Geometry: final body of the model. Coordinates: model frame, mm. Face numbers are marked on the shaded views. A direction names the side the tool comes from. Coordinates: 2 decimals unless noted, no trailing zeros. Loops run counter-clockwise (first coordinate to the right, second up) from the corner with the lowest first, then second, coordinate; pieces in that order, holes last. Notation, with made-up numbers: (74.5, 46) -> (111.5, 46) arc R21 cw to (111.5, 51) -> close; hole circle Ø9 at (28, -8). An arc over 180 degrees is marked (long way). One line per item, written item: value. Start each with the question number.
Item 1: Section query A-A on y = -14. Return loops of the section in (x, z), then the cut area to 3 significant figures.
Item 2: Section query C-C on z = 11.5. Return loops of the section in (x, y).
Item 3: Ray query, probe 1 along Y at (x, z) = (0, 1); probe 2 along Z at (x, y) = (-55.5, -6.5); probe 3 along Y at (x, z) = (0, 27). Return the intervals inside material, ascending. Write a range as from..to.
Item 4: Section query D-D on z = 34.5. Return loops of the section in (x, y), then the cut area to 3 significant figures.
Item 5: Mould query, pull axis Y, two halves, no side actions, for the marked faces 1, 2, 3 and 4. Classes: +Y half, -Y half, draft (parallel to the pull), parting line (faces both ways), or undercut.
Item 6: Set-up query: the marked faces 5, 6 and 7. Return all of +Z, -Z, +X, -X, +Y, -Y with unobstructed straight access to the full face (end or side cutting, diameter ignored); none if empty.
Item 7: Section query B-B on x = -10.5. Return loops of the section in (y, z).
Item 8: Contact query for flat-ended pins moving along their axis: pin 1 Ø12 at (y, z) = (-17, 18.5) entering from +X; pin 2 Ø19.5 at (x, z) = (-60, 18) entering from -Y; pin 3 Ø12 at (x, y) = (50, -44.5) entering from +Z; pin 4 Ø7.5 at (x, z) = (59, 16) entering from -Y. Output: stop coordinate, or through.
from build123d import *

# Parameters (mm, degrees)
F0_R      = 67.5
F1_DEPTH  = 3
F2_R      = 43
F2_R_2    = 41
F3_DEPTH  = 35
F4_R      = 27.5
F5_DEPTH  = 3
F7_DEPTH  = 25
F12_DEPTH = 25
F13_DEPTH = 25
F14_DEPTH = 25
F15_DEPTH = 25
F16_DEPTH = 25


with BuildPart() as f1:
    # F0 (on Top) → F1 (new body)
    with BuildSketch(Plane.XY):
        Circle(F0_R)
    extrude(amount=F1_DEPTH)

    # F2 (on face) → F3 (join)
    with BuildSketch(Plane.XY.offset(3)):
        Circle(F2_R)
        Circle(F2_R_2, mode=Mode.SUBTRACT)
    extrude(amount=F3_DEPTH)

    # F4 (on face) → F5 (cut)
    with BuildSketch(Plane.XY.offset(3)):
        Circle(F4_R)
    extrude(amount=-F5_DEPTH, mode=Mode.SUBTRACT)

    # F6 (on face) → F7 (join)
    with BuildSketch(Plane.XY.offset(3)):
        with BuildLine():
            ThreePointArc((-1.4872706737, -67.4836130179), (0.0127324705, -67.4999987991), (1.5127293263, -67.4830471303))
            Line((1.5127293263, -67.4830471303), (1.5127293263, -42.973383041))
            ThreePointArc((1.5127293263, -42.973383041), (0.0127370783, -42.9999981136), (-1.4872706737, -42.9742716744))
            Line((-1.4872706737, -42.9742716744), (-1.4872706737, -67.4836130179))
        make_face()
        with BuildLine():
            Line((67.4833312752, -1.5), (67.4833312752, 1.5))
            Line((67.4833312752, 1.5), (42.9738292453, 1.5))
            ThreePointArc((42.9738292453, 1.5), (42.9934568135, 0.7501141427), (43, 0))
            ThreePointArc((43, 0), (42.9934568135, -0.7501141427), (42.9738292453, -1.5))
            Line((42.9738292453, -1.5), (67.4833312752, -1.5))
        make_face()
        with BuildLine():
            Line((-42.9738292453, 1.5), (-67.4833312752, 1.5))
            Line((-67.4833312752, 1.5), (-67.4833312752, -1.5))
            Line((-67.4833312752, -1.5), (-42.9738292453, -1.5))
            ThreePointArc((-42.9738292453, -1.5), (-43, 0), (-42.9738292453, 1.5))
        make_face()
        with BuildLine():
            ThreePointArc((1.5, 67.4833312752), (0.7500463063, 67.4958326902), (0, 67.5))
            ThreePointArc((0, 67.5), (-0.7500463063, 67.4958326902), (-1.5, 67.4833312752))
            Line((-1.5, 67.4833312752), (-1.5, 42.9738292453))
            ThreePointArc((-1.5, 42.9738292453), (0, 43), (1.5, 42.9738292453))
            Line((1.5, 42.9738292453), (1.5, 67.4833312752))
        make_face()
    extrude(amount=F7_DEPTH)

    # F11 (on face) → F12 (cut)
    with BuildSketch(Plane.YZ.offset(1.5127293263)):
        with BuildLine():
            Line((-67.4830471303, 28), (-67.4830471303, 3))
            ThreePointArc((-67.4830471303, 3), (-52.1775932535, 12.5092113453), (-42.973383041, 28))
            Line((-42.973383041, 28), (-67.4830471303, 28))
        make_face()
    extrude(amount=-F12_DEPTH, mode=Mode.SUBTRACT)

    # F8 (on face) → F13 (cut)
    with BuildSketch(Plane(origin=(0, 1.5, 0), x_dir=(-1, 0, 0), z_dir=(0, 1, 0))):
        with BuildLine():
            Line((-67.4833312752, 28), (-67.4833312752, 3))
            ThreePointArc((-67.4833312752, 3), (-52.177969566, 12.5092420399), (-42.9738292453, 28))
            Line((-42.9738292453, 28), (-67.4833312752, 28))
        make_face()
    extrude(amount=-F13_DEPTH, mode=Mode.SUBTRACT)

    # F9 (on face) → F14 (cut)
    with BuildSketch(Plane(origin=(-1.5, 0, 0), x_dir=(0, -1, 0), z_dir=(-1, 0, 0))):
        with BuildLine():
            Line((-67.4833312752, 28), (-67.4833312752, 3))
            ThreePointArc((-67.4833312752, 3), (-52.177969566, 12.5092420399), (-42.9738292453, 28))
            Line((-42.9738292453, 28), (-67.4833312752, 28))
        make_face()
    extrude(amount=-F14_DEPTH, mode=Mode.SUBTRACT)

    # F10 (on face) → F15 (cut)
    with BuildSketch(Plane.XZ.offset(1.5)):
        with BuildLine():
            Line((-67.4833312752, 28), (-67.4833312752, 3))
            ThreePointArc((-67.4833312752, 3), (-52.177969566, 12.5092420399), (-42.9738292453, 28))
            Line((-42.9738292453, 28), (-67.4833312752, 28))
        make_face()
    extrude(amount=-F15_DEPTH, mode=Mode.SUBTRACT)

    # F16 (cut, through all): faces of the model
    f16_faces = [f1.faces().sort_by_distance(p)[0] for p in [
        (0, 67.4899988357, 28),
        (0.0003160568, -67.4898297441, 28),
        (0, 67.4899988357, 28),
        (0.0003160568, -67.4898297441, 28),
    ]]
    extrude(f16_faces, amount=-F16_DEPTH, mode=Mode.SUBTRACT)


solid = f1.part
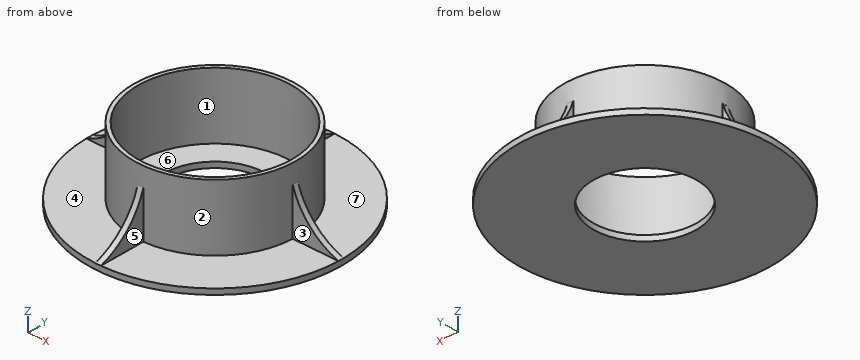
Reply:
1. outline: (-66.03, 0) -> (-23.67, 0) -> (-23.67, 3) -> (-38.54, 3) -> (-38.54, 38) -> (-40.66, 38) -> (-40.66, 3) -> (-66.03, 3) -> close; (23.67, 0) -> (66.03, 0) -> (66.03, 3) -> (40.66, 3) -> (40.66, 38) -> (38.54, 38) -> (38.54, 3) -> (23.67, 3) -> close
1. area: 403 mm²
2. outline: (-53.21, -1.5) -> (-42.97, -1.5) arc R43 ccw to (-1.49, -42.97) -> (-1.49, -53.21) -> (1.51, -53.21) -> (1.51, -42.97) arc R43 ccw to (42.97, -1.5) -> (53.21, -1.5) -> (53.21, 1.5) -> (42.97, 1.5) arc R43 ccw to (1.5, 42.97) -> (1.5, 53.21) -> (-1.5, 53.21) -> (-1.5, 42.97) arc R43 ccw to (-42.97, 1.5) -> (-53.21, 1.5) -> close; hole circle Ø82 at (0, 0)
3. probe 1: y = -67.5..-27.5, 27.5..67.5
3. probe 2: z = 0..3
3. probe 3: y = -43.29..-41, 41..43.29
4. outline: circle Ø86 at (0, 0); hole circle Ø82 at (0, 0)
4. area: 528 mm²
5. face 1: undercut
5. face 2: parting line
5. face 3: -Y half
5. face 4: draft
6. face 5: +Z, +X, -Y
6. face 6: +Z
6. face 7: +Z, +X, +Y
7. outline: (-66.68, 0) -> (-25.42, 0) -> (-25.42, 3) -> (-39.63, 3) -> (-39.63, 38) -> (-41.7, 38) -> (-41.7, 3) -> (-66.68, 3) -> close; (25.42, 0) -> (66.68, 0) -> (66.68, 3) -> (41.7, 3) -> (41.7, 38) -> (39.63, 38) -> (39.63, 3) -> (25.42, 3) -> close
8. pin 1: stops at x = 41.57
8. pin 2: stops at y = -1.5
8. pin 3: stops at z = 3
8. pin 4: passes through
